The drawing under review shows one solid part. Ordinate dimensions are in mm from its lowest x, y, z. Give positions to 0.01 mm unless a question says otherwise; leave off trailing zeros. Loops run counter-clockwise (first coordinate to the right, second up) from the corner with the lowest first, then second, coordinate; pieces in that order, holes last. Notation, with made-up numbers: M 11.5,66.25 L 56.5,66.25 A20 ccw 56.5,100.25 Z; hole C 34,84.25 d6. An arc over 180 degrees is marked long. Write item = value, one per line. Start each with the question number.
1. We need section C-C on z = 50. Give the boundary of the cut face in (x, y), then the cut area to 3 significant figures.
2. We need section B-B on y = 35. Give the boundary of the cut face in (x, z).
3. For pin 1 (4 mm diameter, centred on x = 13, z = 77.5, fed in from +Y) (3 decimals); pin 2 (2 mm diameter, centred on y = 24.5, z = 43.5, fed in from -X), all flat-tipped, find the tip position at first contact; note any pin that passes through.
4. Wall thickness on line 1 along Y through (x, z) = (32.5, 50); line 2 along Z through (x, y) = (43.5, 8.5); line 3 along Y through (x, z) = (4.5, 33): over which ranges is each line inside the solid? List them lowest first. Write a range as from..to.
5. We need section D-D on x = 39.5. Give the boundary of the cut face in (y, z), then the cut area to 3 significant figures.
6. We need section A-A on z = 72. Give the boundary of the cut face in (x, y), then the cut area to 3 significant figures.
7. Draft analysis for pull direction Y (two halves, no side actions). For the marked faces 1, 2 and 3, state which applies: pulls with the +Y half, pulls with the -Y half, needs draft (parallel to the pull), parting line crosses it, or undercut.
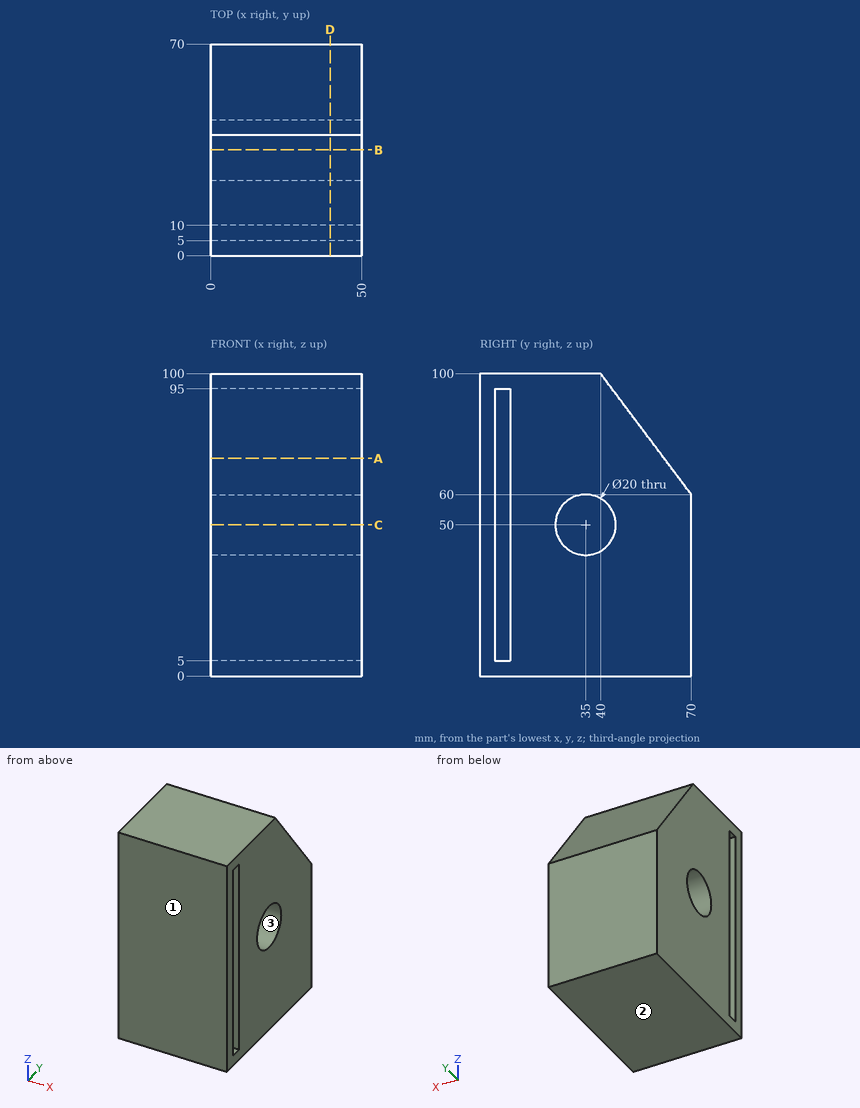
Final values:
q1.outline = M 0,0 L 50,0 L 50,5 L 0,5 Z; M 0,10 L 50,10 L 50,25 L 0,25 Z; M 0,45 L 50,45 L 50,70 L 0,70 Z
q1.area = 2,250 mm²
q2.outline = M 0,0 L 50,0 L 50,40 L 0,40 Z; M 0,60 L 50,60 L 50,100 L 0,100 Z
q3.pin_1 = 58.375
q3.pin_2 = 0
q4.line_1 = 0..5, 10..25, 45..70
q4.line_2 = 0..5, 95..100
q4.line_3 = 0..5, 10..70
q5.outline = M 0,0 L 70,0 L 70,60 L 40,100 L 0,100 Z; hole M 5,5 L 10,5 L 10,95 L 5,95 Z; hole C 35,50 d20
q5.area = 5,640 mm²
q6.outline = M 0,0 L 50,0 L 50,5 L 0,5 Z; M 0,10 L 50,10 L 50,61 L 0,61 Z
q6.area = 2,800 mm²
q7.face_1 = pulls with the -Y half
q7.face_2 = needs draft
q7.face_3 = undercut
